```python
from build123d import *

# Parameters (mm, degrees)
F1_DEPTH = 166
F3_DEPTH = 2
F4_D     = 20
F4_DEPTH = 5


with BuildPart() as f1:
    # F0 (on Front) → F1 (new body)
    with BuildSketch(Plane.XZ):
        with BuildLine():
            ThreePointArc((0, 12), (0.585786, 10.585786), (2, 10))
            Line((2, 10), (408, 10))
            ThreePointArc((408, 10), (409.414214, 10.585786), (410, 12))
            Line((410, 12), (410, 20))
            Line((410, 20), (408, 20))
            Line((408, 20), (408, 12))
            Line((408, 12), (2, 12))
            Line((2, 12), (2, 20))
            Line((2, 20), (0, 20))
            Line((0, 20), (0, 12))
        make_face()
    extrude(amount=-F1_DEPTH)

    # F2 (on face) → F3 (cut, through all)
    with BuildSketch(Plane(origin=(0, 0, 10), x_dir=(1, 0, 0), z_dir=(0, 0, -1))):
        with BuildLine():
            ThreePointArc((310, -20), (300, -10), (290, -20))
            Line((290, -20), (290, -105))
            ThreePointArc((290, -105), (300, -115), (310, -105))
            Line((310, -105), (310, -20))
        make_face()
        with BuildLine():
            ThreePointArc((350, -20), (340, -10), (330, -20))
            Line((330, -20), (330, -105))
            ThreePointArc((330, -105), (340, -115), (350, -105))
            Line((350, -105), (350, -20))
        make_face()
        with BuildLine():
            ThreePointArc((390, -20), (380, -10), (370, -20))
            Line((370, -20), (370, -105))
            ThreePointArc((370, -105), (380, -115), (390, -105))
            Line((390, -105), (390, -20))
        make_face()
    extrude(amount=-F3_DEPTH, mode=Mode.SUBTRACT)

    # F4
    with Locations(Plane(origin=(0, 0, 10), x_dir=(1, 0, 0), z_dir=(0, 0, -1))):
        with Locations((300, -166), (340, -166), (380, -166)):
            Hole(F4_D / 2, depth=F4_DEPTH)


solid = f1.part
```
Check sheet for the modelled part. Datum: model origin and axes. Units: mm. A direction names the side the tool comes from. Round coordinates to 2 decimals unless told otherwise and drop trailing zeros. Order: outer loops, then holes, each group sorted by start corner. A loop starts at its lowest first (then second) coordinate and runs counter-clockwise, first axis right, second up.
1) Section check B-B (y = 84). Record the boundary of the cut face in (x, z).
2) Section check D-D (y = 140). Record the boundary of the cut face in (x, z), and give its area (3 significant figures).
3) Tool access check on faces 4 (the cylindrical face through (380, 115, 11)), 5 (the cylindrical face through (300, 156, 11)), 6 (the flat face through (2, 82, 16)). Record the directions out of +Z, -Z, +X, -X, +Y, -Y that give a thin tool (end or side, any length) a straight path to the whole face; none if there is none.
4) Scan lines: line 1 (X direction, y = 78, z = 11.5); line 2 (X direction, y = 116.5, z = 15); line 3 (Z direction, x = 223, y = 77). Record each from-to range of solid material in increasing order.
5) Mould release check, pull along X, two halves, no side actions. Record for faces 1 (the flat face through (402.2, 166, 11.7)), 2 (the flat face through (410, 82, 16)), 3 (the cylindrical face through (380, 156, 11)): +X half, -X half, draft (parallel to the pull), parting line (faces both ways), or undercut.
6) Section check A-A (x = 300). Record the boundary of the cut face in (y, z).
7) Section check C-C (z = 18). Record the boundary of the cut face in (x, y), and give its area (3 significant figures).
8) Go/stop test with flat-tipped pins: pin 1 Ø1.6 at (y, z) = (42.5, 10.5) entering from -X; pin 2 Ø1 at (y, z) = (52, 10.5) entering from +X; pin 3 Ø1 at (y, z) = (44.5, 10.5) entering from -X. Record where each tip stops, or that it passes through.
Result:
1. outline: (0, 12) arc R2 ccw to (2, 10) - (290, 10) - (290, 12) - (2, 12) - (2, 20) - (0, 20) - close; (310, 10) - (330, 10) - (330, 12) - (310, 12) - close; (350, 10) - (370, 10) - (370, 12) - (350, 12) - close; (390, 10) - (408, 10) arc R2 ccw to (410, 12) - (410, 20) - (408, 20) - (408, 12) - (390, 12) - close
2. outline: (0, 12) arc R2 ccw to (2, 10) - (408, 10) arc R2 ccw to (410, 12) - (410, 20) - (408, 20) - (408, 12) - (2, 12) - (2, 20) - (0, 20) - close
2. area: 850 mm2
3. face 4: +Z, -Z
3. face 5: +Z, -Z, +Y
3. face 6: +Z, +Y, -Y
4. line 1: x = 0.06 to 290, 310 to 330, 350 to 370, 390 to 409.94
4. line 2: x = 0 to 2, 408 to 410
4. line 3: z = 10 to 12
5. face 1: draft
5. face 2: +X half
5. face 3: undercut
6. outline: (0, 10) - (10, 10) - (10, 12) - (0, 12) - close; (115, 10) - (156, 10) - (156, 12) - (115, 12) - close
7. outline: (0, 0) - (2, 0) - (2, 166) - (0, 166) - close; (408, 0) - (410, 0) - (410, 166) - (408, 166) - close
7. area: 664 mm2
8. pin 1: stops at x = 0.13
8. pin 2: stops at x = 409.73
8. pin 3: stops at x = 0.27
